Answer from the drawing. Dimensions are ordinates in mm from the lowest x, y and z of the part. Coordinates: 2 decimals unless noted, no trailing zeros. Write each loop counter-clockwise with the first axis right and the second up, starting at its lowest first coordinate (ties: lowest second). Pieces come first, ordered by that corner, then holes. Notation, with made-up numbers: (37.5, -14.5) - (82.5, -14.5) arc R15 cw to (82.5, -6.5) - close; hole circle Ø6 at (6.25, -1). An arc over 180 degrees is marked (long way). Return JSON: item names as keys, results as strings.
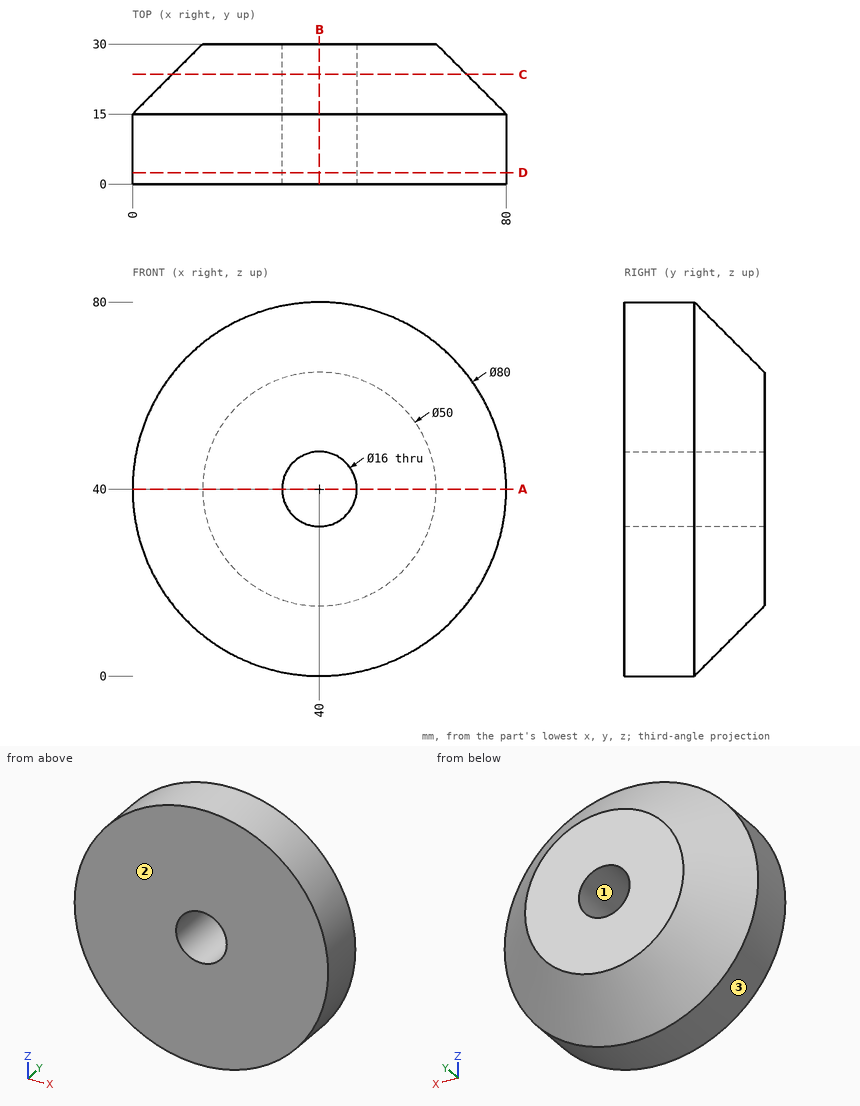
(1) Determine the mould class of the marked faces 1, 2 and 3 for opening direction Z: +Z half, -Z half, draft (parallel to the pull), parting line (faces both ways), or undercut.
Answer:
{"face 1": "undercut", "face 2": "draft", "face 3": "parting line"}
(2) Straight lines are drawn through the part: line 1 (Z direction, x = 40, y = 8.75); line 2 (Z direction, x = 35, y = 28.5) (3 decimals); line 3 (Y direction, x = 23.5, z = 16.5). For each, find the intervals that lie inside material, in ascending order. Write a range as from..to.
Answer:
{"line 1": "0..32, 48..80", "line 2": "13.976..33.755, 46.245..66.024", "line 3": "0..26.29"}
(3) A cutting plane is placed at B-B (x = 40). Determine the outline of the cut face in (y, z).
Answer:
{"outline": "(0, 0) - (15, 0) - (30, 15) - (30, 32) - (0, 32) - close; (0, 48) - (30, 48) - (30, 65) - (15, 80) - (0, 80) - close"}
(4) Flat-ended cylindrical pins translate along their axes: P1, Ø1, axis at y = 18.5, z = 68.5, coming from the -X side; P2, Ø4, axis at y = 4.5, z = 20, coming from the +X side; P3, Ø10, axis at x = 65.5, y = 8.5, coming from the +Z side. Find the tip coordinate at first contact, or state that the pin passes through.
Answer:
{"P1": "x = 16.2", "P2": "x = 75.72", "P3": "z = 74.35"}
(5) A cutting plane is placed at D-D (y = 2.5). Determine the outline of the cut face in (x, z).
Answer:
{"outline": "circle Ø80 at (40, 40); hole circle Ø16 at (40, 40)"}
(6) A cutting plane is placed at C-C (y = 23.5). Determine the outline of the cut face in (x, z), and give its area (3 significant figures).
Answer:
{"outline": "circle Ø63 at (40, 40); hole circle Ø16 at (40, 40)", "area": "2,920 mm²"}
(7) A cutting plane is placed at A-A (z = 40). Determine the outline of the cut face in (x, y).
Answer:
{"outline": "(0, 0) - (32, 0) - (32, 30) - (15, 30) - (0, 15) - close; (48, 0) - (80, 0) - (80, 15) - (65, 30) - (48, 30) - close"}
